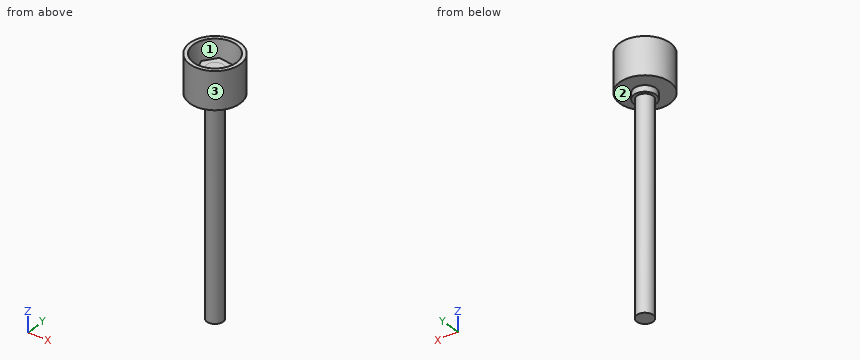
from build123d import *

# Parameters (mm, degrees)
F0_R          = 5.5245
F1_DEPTH      = 20.32
F1_DEPTH_BACK = 141.859
F2_R          = 7.4676
F2_R_2        = 5.5245
F3_DEPTH      = 4.2418
F4_R          = 17.145
F5_DEPTH      = 5.08
F7_DEPTH      = 10.8712
F8_R          = 17.145
F8_R_2        = 14.605
F9_DEPTH      = 20.32


with BuildPart() as f1:
    # F0 (on Top) → F1 (new body, two sides)
    with BuildSketch(Plane.XY) as f1_sk:
        Circle(F0_R)
    extrude(amount=F1_DEPTH)
    extrude(f1_sk.sketch, amount=-F1_DEPTH_BACK)

    # F2 (on Top) → F3 (join)
    with BuildSketch(Plane.XY):
        Circle(F2_R)
        Circle(F2_R_2, mode=Mode.SUBTRACT)
    extrude(amount=F3_DEPTH)

    # F4 (on face) → F5 (join)
    with BuildSketch(Plane.XY.offset(4.2418)):
        Circle(F4_R)
    extrude(amount=F5_DEPTH)

    # F6 (on face) → F7 (join)
    with BuildSketch(Plane.XY.offset(9.3218)):
        Polygon((4.207769, -9.34719), (10.198788, -1.02956), (5.991019, 8.31763), (-4.207769, 9.34719), (-10.198788, 1.02956), (-5.991019, -8.31763), align=None)
    extrude(amount=F7_DEPTH)

    # F8 (on face) → F9 (join)
    with BuildSketch(Plane.XY.offset(9.3218)):
        Circle(F8_R)
        Circle(F8_R_2, mode=Mode.SUBTRACT)
    extrude(amount=F9_DEPTH)

    # F10 (on Right) → F11 (revolve)
    with BuildSketch(Plane.YZ):
        Polygon((-14.605, 29.6418), (-14.605, 9.3218), (-12.065, 9.3218), align=None)
    revolve(axis=Axis((0, 0, 15.219002), (0, 0, 1)))


solid = f1.part
Here's how the part is built. I have some questions about the finished solid (model axes, mm). Face numbers are marked on the shaded views. Give positions to 0.01 mm unless a question says otherwise; leave off trailing zeros. Order: outer loops, then holes, each group sorted by start corner. A loop starts at its lowest first (then second) coordinate and runs counter-clockwise, first axis right, second up. Notation, with made-up numbers: (9, 77.25) -> (14, 77.25) arc R26 cw to (14, 91.25) -> close; hole circle Ø11 at (39, -29.75). An arc over 180 degrees is marked (long way). One line per item, written item: value. Start each with the question number.
1. Will these pins go through, and if not, where does the flat tip stop? pin 1 Ø4 at (x, z) = (9.5, -86.5) entering from +Y; pin 2 Ø12 at (x, y) = (1.5, -4) entering from +Z; pin 3 Ø4 at (x, z) = (1.5, -90.5) entering from +Y; pin 4 Ø4 at (x, y) = (-10, 2.5) entering from -Z.
2. I need wall thicknesses on probe 1 along Z at (x, y) = (14, -8.5); probe 2 along X at (y, z) = (-3.5, 19.5); probe 3 along Z at (x, y) = (-2, -5.5). Which ranges of each line are inside material? Lowest first, please. Write a range as from..to.
3. Imagine slicing it at B-B, the plane z = -97.5. List the corners of the cut face in (x, y) for me.
4. Imagine slicing it at A-A, the plane z = 15.5. List the corners of the cut face in (x, y) for me (3 decimals), plus the area to 3 significant figures.
5. We'd pull the mould along Y, two halves only. Please class the marked faces 1, 2 and 3: released by +Y, released by -Y, zero draft, split by the parting line, or undercut.
Values follow:
1. pin 1: passes through
1. pin 2: stops at z = 20.32
1. pin 3: stops at y = 5.52
1. pin 4: stops at z = 4.24
2. probe 1: z = 4.24..29.64
2. probe 2: x = -16.78..-12.87, -8.16..8.42, 12.87..16.78
2. probe 3: z = 0..20.19
3. outline: circle Ø11.05 at (0, 0)
4. outline: circle Ø34.29 at (0, 0); (-10.199, 1.03) -> (-5.991, -8.318) -> (4.208, -9.347) -> (10.199, -1.03) -> (5.991, 8.318) -> (-4.208, 9.347) -> close; hole circle Ø25.675 at (0, 0)
4. area: 679 mm2
5. face 1: undercut
5. face 2: zero draft
5. face 3: split by the parting line
